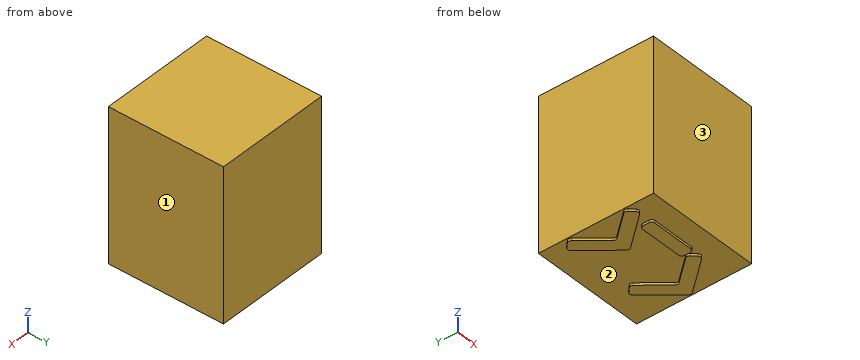
from build123d import *

# Parameters (mm, degrees)
SKETCH_W            = 19
SKETCH_H            = 19
PAD_DEPTH           = 25
PAD001_DEPTH        = 0.4
LINEARPATTERN_COUNT = 2
LINEARPATTERN_PITCH = 12
PAD002_DEPTH        = 0.4


with BuildPart() as part:
    # Sketch → Pad (new body)
    with BuildSketch(Plane.XY):
        Rectangle(SKETCH_W, SKETCH_H)
    extrude(amount=PAD_DEPTH)

    # Sketch001 → Pad001 (join)
    with BuildSketch(Plane.XY):
        with BuildLine():
            Line((-9.183343, 4.331109), (-5.818792, 0.321394))
            ThreePointArc((-5.818792, -0.321394), (-5.701815, 0), (-5.818792, 0.321394))
            Line((-5.818792, -0.321394), (-9.183343, -4.331109))
            ThreePointArc((-9.183343, -4.331109), (-9.299845, -4.674313), (-9.153874, -5.006057))
            Line((-9.153874, -5.006057), (-8.444067, -5.715864))
            ThreePointArc((-8.444067, -5.715864), (-8.068704, -5.861835), (-7.707491, -5.683705))
            Line((-7.707491, -5.683705), (-3.207978, -0.321394))
            ThreePointArc((-3.207978, -0.321394), (-3.091, 0), (-3.207978, 0.321394))
            Line((-3.207978, 0.321394), (-7.707491, 5.683705))
            ThreePointArc((-7.707491, 5.683705), (-8.068704, 5.861835), (-8.444067, 5.715864))
            Line((-8.444067, 5.715864), (-9.153874, 5.006057))
            ThreePointArc((-9.153874, 5.006057), (-9.299845, 4.674313), (-9.183343, 4.331109))
        make_face()
    pad001 = extrude(amount=-PAD001_DEPTH)

    # LinearPattern: Pad001 ×2
    with Locations(*[(i * LINEARPATTERN_PITCH, 0, 0) for i in range(1, LINEARPATTERN_COUNT)]):
        add(pad001)

    # Sketch002 → Pad002 (join)
    with BuildSketch(Plane(origin=(0, 0, 0), x_dir=(1, 0, 0), z_dir=(0, 0, -1))):
        with BuildLine():
            ThreePointArc((-5.15, 6), (-5.503553, 5.853553), (-5.65, 5.5))
            Line((-5.65, 4.5), (-5.65, 5.5))
            ThreePointArc((-5.65, 4.5), (-5.503553, 4.146447), (-5.15, 4))
            Line((1.85, 4), (-5.15, 4))
            ThreePointArc((1.85, 4), (2.203553, 4.146447), (2.35, 4.5))
            Line((2.35, 5.5), (2.35, 4.5))
            ThreePointArc((2.35, 5.5), (2.203553, 5.853553), (1.85, 6))
            Line((-5.15, 6), (1.85, 6))
        make_face()
    extrude(amount=PAD002_DEPTH)


solid = part.part
Design review of the part built by this model. Coordinates are the model's own, in mm. Face numbers are marked on the shaded views. Coordinates: 2 decimals unless noted, no trailing zeros. Loops run counter-clockwise (first coordinate to the right, second up) from the corner with the lowest first, then second, coordinate; pieces in that order, holes last. Notation, with made-up numbers: M 77.25,52 L 115.25,52 A11 cw 115.25,72 Z; hole C -12,52 d1. An arc over 180 degrees is marked long. Use one line per item in the form item = value.
(1) Draft analysis for pull direction Y (two halves, no side actions). For the marked faces 1, 2 and 3, state which applies: pulls with the +Y half, pulls with the -Y half, needs draft (parallel to the pull), parting line crosses it, or undercut.
Return value:
face_1 = needs draft
face_2 = undercut
face_3 = pulls with the -Y half
(2) Consider section A-A (y = 8). Write out the cut boundary in (x, z), and give its area (3 significant figures).
Return value:
outline = M -9.5,0 L 9.5,0 L 9.5,25 L -9.5,25 Z
area = 475 mm2
(3) For line 1 along Z through (x, y) = (-7.25, 0.25), list the stretches that pass through material, from the lowest coordinate up. Write a range as from..to.
Return value:
line_1 = 0..25
